from build123d import *

# Parameters (mm, degrees)
CROQUIS1_W                                           = 360
CROQUIS1_H                                           = 80
SALIENTE_EXTRUIR1_DEPTH                              = 15
CROQUIS2_W                                           = 360
CROQUIS2_H                                           = 80
CROQUIS2_W_2                                         = 330
CROQUIS2_H_2                                         = 56
CORTAR_EXTRUIR1_DEPTH                                = 2
REFRENTADO_PARA_TORNILLO_CON_CABEZA_HUEC_D           = 4.5
REFRENTADO_PARA_TORNILLO_CON_CABEZA_HUEC_CBORE_D     = 8
REFRENTADO_PARA_TORNILLO_CON_CABEZA_HUEC_CBORE_DEPTH = 4.4
TALADROS_DE_ESPIGA_DE_4_0MM1_D                       = 4
TALADRO_ROSCADO_M3X0_351_D                           = 2.65
TALADRO_ROSCADO_M3X0_351_DEPTH                       = 7.75
TALADRO_ROSCADO_M3X0_351_TIP                         = 0.79614032
MATRIZL1_COUNT                                       = 13
MATRIZL1_PITCH                                       = 25
MATRIZL1_COUNT_DIR2                                  = 2
MATRIZL1_PITCH_DIR2                                  = 68


with BuildPart() as part:
    # Croquis1 → Saliente-Extruir1 (new body)
    with BuildSketch(Plane.XY):
        with Locations((180, 40)):
            Rectangle(CROQUIS1_W, CROQUIS1_H)
    extrude(amount=SALIENTE_EXTRUIR1_DEPTH)

    # Croquis2 → Cortar-Extruir1 (cut)
    with BuildSketch(Plane.XY.offset(15)):
        with Locations((180, 40)):
            Rectangle(CROQUIS2_W, CROQUIS2_H)
        with Locations((180, 40)):
            Rectangle(CROQUIS2_W_2, CROQUIS2_H_2, mode=Mode.SUBTRACT)
    extrude(amount=-CORTAR_EXTRUIR1_DEPTH, mode=Mode.SUBTRACT)

    # Croquis4 → Taladro roscado M31 (revolve, cut)
    with BuildSketch(Plane(origin=(30, 6, 13), x_dir=(0, -1, 0), z_dir=(1, 0, 0))):
        Polygon((0, 0), (0, 7.751075774), (1.25, 7), (1.25, 0), align=None)
    taladro_roscado_m31 = revolve(axis=Axis((30, 6, 19.35), (0, 0, -1)), mode=Mode.SUBTRACT)

    # Refrentado para tornillo con cabeza hueca de M41 (through all)
    with Locations(Plane(origin=(0, 0, 0), x_dir=(-1, 0, 0), z_dir=(0, 0, -1))):
        with Locations((-6, 72), (-6, 8), (-354, 72), (-354, 8), (-354, 51), (-354, 29), (-6, 51), (-6, 29)):
            CounterBoreHole(REFRENTADO_PARA_TORNILLO_CON_CABEZA_HUEC_D / 2, REFRENTADO_PARA_TORNILLO_CON_CABEZA_HUEC_CBORE_D / 2, REFRENTADO_PARA_TORNILLO_CON_CABEZA_HUEC_CBORE_DEPTH)

    # Taladros de espiga de Ø4.0mm1 (through all)
    with Locations(Plane(origin=(0, 0, 0), x_dir=(-1, 0, 0), z_dir=(0, 0, -1))):
        with Locations((-6, 64), (-6, 16), (-354, 64), (-354, 16)):
            Hole(TALADROS_DE_ESPIGA_DE_4_0MM1_D / 2)

    # Taladro roscado M3x0.351
    with Locations(Plane(origin=(0, 0, 0), x_dir=(-1, 0, 0), z_dir=(0, 0, -1))):
        with Locations((-21, 73.5), (-51, 73.5), (-51, 6.5), (-21, 6.5)):
            Hole(TALADRO_ROSCADO_M3X0_351_D / 2, depth=TALADRO_ROSCADO_M3X0_351_DEPTH)
            with Locations((0, 0, -(TALADRO_ROSCADO_M3X0_351_DEPTH + TALADRO_ROSCADO_M3X0_351_TIP / 2))):  # 118° drill point
                Cone(0, TALADRO_ROSCADO_M3X0_351_D / 2, TALADRO_ROSCADO_M3X0_351_TIP, mode=Mode.SUBTRACT)

    # MatrizL1: Taladro roscado M31 13 × 2
    with Locations(*[(i * MATRIZL1_PITCH, j * MATRIZL1_PITCH_DIR2, 0) for i in range(MATRIZL1_COUNT) for j in range(MATRIZL1_COUNT_DIR2) if (i, j) != (0, 0)]):
        add(taladro_roscado_m31, mode=Mode.SUBTRACT)


solid = part.part
CAD build for the part. Positions are in the model's coordinates, mm. A direction names the side the tool comes from. Round coordinates to 2 decimals unless told otherwise and drop trailing zeros. Write each loop counter-clockwise with the first axis right and the second up, starting at its lowest first coordinate (ties: lowest second). Pieces come first, ordered by that corner, then holes. Notation, with made-up numbers: M 73,59.25 L 80,59.25 A30 ccw 80,96.25 Z; hole C 55.25,14.25 d5. An arc over 180 degrees is marked long. Use a Markdown table: item, result. Add a question column.
1. Slice it at A-A on x = 40.5. Give the cut face in (y, z).
2. 3-axis set-ups, long thin cutter, end or side, ignore diameter. For faces 1 (the face through (4, 27, 4.4)), 2 (the face through (177, 80, 6)): which of +Z, -Z, +X, -X, +Y, -Y reach the whole face in a straight line?
3. Pull direction X, two halves, no side cores. Call faces 3 (the face through (358, 29, 2)), 4 (the face through (179, 11, 13)), 5 (the face through (0, 39, 6)): released by +X, released by -X, zero draft, split by the parting line, or undercut.
4. Drill centre lines: probe 1 along Y at (x, z) = (105, 11.75); probe 2 along X at (y, z) = (73.5, 5.25) (3 decimals); probe 3 along X at (y, z) = (17.5, 10.5). Where is each one in solid material? Low to high.
5. Flat gauge pins, fed straight in: P1, Ø4, axis at x = 112.5, z = 8.5, coming from the -Y side; P2, Ø2, axis at x = 30, y = 6, coming from the +Z side; P3, Ø1.6, axis at x = 166, z = 14.5, coming from the -Y side. Where does each tip first touch, or does it go through?
Reply:
| question | item | result |
|---|---|---|
| 1 | outline | M 0,0 L 80,0 L 80,13 L 68,13 L 68,15 L 12,15 L 12,13 L 0,13 Z |
| 2 | face 1 | -Z |
| 2 | face 2 | +Z, -Z, +X, -X, +Y |
| 3 | face 3 | undercut |
| 3 | face 4 | zero draft |
| 3 | face 5 | released by -X |
| 4 | probe 1 | y = 0 to 4.75, 7.25 to 72.75, 75.25 to 80 |
| 4 | probe 2 | x = 0 to 4.323, 7.677 to 19.675, 22.325 to 49.675, 52.325 to 352.323, 355.677 to 360 |
| 4 | probe 3 | x = 0 to 4.68, 7.32 to 352.68, 355.32 to 360 |
| 5 | P1 | stops at y = 0 |
| 5 | P2 | stops at z = 5.85 |
| 5 | P3 | stops at y = 12 |
